Input: part model. Units: mm. Frame: model coordinates. A direction names the side the tool comes from. Coordinates: 2 decimals unless noted, no trailing zeros. Write each loop counter-clockwise with the first axis right and the second up, starting at its lowest first coordinate (ties: lowest second). Pieces come first, ordered by that corner, then holes.
1) Draft query along Z for faces 3 (the cylindrical face through (34.057, -9.392, 21.175)), 4 (the cylindrical face through (-31.902, -9.392, 44.844)), 5 (the flat face through (-1, -19.05, -3)). Return one class per face: pulls with the +Z half, pulls with the -Z half, needs draft (parallel to the pull), parting line crosses it, or undercut.
2) Section query D-D (x = 42.5). Output: boundary loops of the cut face in (y, z).
3) Line query: L1, parallel to X at y = -4, z = 33.5; L2, parallel to X at y = -13.5, z = 35.5; L3, parallel to Z at x = -2, y = -17.75. Output: solid intervals per line, ascending.
4) Set-up query: faces 1 (the cylindrical face through (57.706, -9.392, 4.542)), 2 (the cylindrical face through (-33.183, -9.392, 20.063)). Return all of +Z, -Z, +X, -X, +Y, -Y with unobstructed straight access to the full face (end or side cutting, diameter ignored); none if empty.
5) Section query A-A (z = 30). Output: boundary loops of the cut face in (x, y), then the cut area to 3 significant figures.
6) Section query B-B (y = -2.5). Output: boundary loops of the cut face in (x, z), then the cut area to 3 significant figures.
7) Pin query (flat end, axial travel): pin 1 Ø4 at (x, y) = (-35, -14.5) entering from +Z; pin 2 Ø10 at (x, y) = (-6, -16.5) entering from -Z; pin 3 Ø10 at (x, y) = (4.5, -13) entering from +Z. Return the tip coordinate at first contact, or that it passes through.
8) Section query C-C (z = 16). Output: boundary loops of the cut face in (x, y), then the cut area to 3 significant figures.
from build123d import *

# Parameters (mm, degrees)
F0_W     = 7.112
F0_H     = 7.316239
F1_DEPTH = 19.05


with BuildPart() as f1:
    # F0 (on Front) → F1 (new body)
    with BuildSketch(Plane.XZ):
        with BuildLine():
            ThreePointArc((-27.114501, 38.893752), (-32.012181, 44.876616), (-39.353315, 42.44975))
            ThreePointArc((-39.353315, 42.44975), (-57.738612, 4.113074), (-44.973303, -36.44265))
            ThreePointArc((-44.973303, -36.44265), (0.170855, -20.527097), (45.573682, -35.688993))
            ThreePointArc((45.573682, -35.688993), (57.655342, 5.150357), (38.526372, 43.201659))
            ThreePointArc((38.526372, 43.201659), (30.320612, 46.569585), (26.283572, 38.671501))
            ThreePointArc((26.283572, 38.671501), (34.091174, 20.901024), (30.76575, 1.778))
            Line((30.76575, 1.778), (-14.44625, 1.778))
            Line((-14.44625, 1.778), (-27.14625, 1.778))
            ThreePointArc((-27.14625, 1.778), (-33.184244, 20.341054), (-27.114501, 38.893752))
        make_face()
        with Locations((1.80975, -8.780336)):
            Rectangle(F0_W, F0_H, mode=Mode.SUBTRACT)
        with Locations((1.80975, -8.780336)):
            Rectangle(F0_W, F0_H)
    extrude(amount=F1_DEPTH)


solid = f1.part
Answer:
1. face 3: undercut
1. face 4: pulls with the +Z half
1. face 5: needs draft
2. outline: (-19.05, -33.46) - (0, -33.46) - (0, 39.3) - (-19.05, 39.3) - close
3. L1: x = -47.21 to -30.29, 29.92 to 47.21
3. L2: x = -45.72 to -29.28, 28.68 to 45.72
3. L3: z = -20.58 to 1.78
4. face 1: +X, +Y, -Y
4. face 2: +Y, -Y
5. outline: (-49.5, -19.05) - (-31.66, -19.05) - (-31.66, 0) - (-49.5, 0) - close; (31.66, -19.05) - (49.5, -19.05) - (49.5, 0) - (31.66, 0) - close
5. area: 680 mm2
6. outline: (-44.97, -36.44) arc R73.73 cw to (45.57, -35.69) arc R57.88 ccw to (38.53, 43.2) arc R6.55 ccw to (26.28, 38.67) arc R33.59 cw to (30.77, 1.78) - (-27.15, 1.78) arc R31.47 cw to (-27.11, 38.89) arc R6.83 ccw to (-39.35, 42.45) arc R57.88 ccw to start
6. area: 4,870 mm2
7. pin 1: stops at z = 45.15
7. pin 2: stops at z = -21.47
7. pin 3: stops at z = 1.78
8. outline: (-55.63, -19.05) - (-32.89, -19.05) - (-32.89, 0) - (-55.63, 0) - close; (34.33, -19.05) - (55.63, -19.05) - (55.63, 0) - (34.33, 0) - close
8. area: 839 mm2
